from build123d import *

# Parameters (mm, degrees)
SKETCH1_W                 = 12
SKETCH1_H                 = 12
BOSS_EXTRUDE1_DEPTH       = 2
SKETCH2_W                 = 2.5
SKETCH2_H                 = 12
BOSS_EXTRUDE2_DEPTH       = 8
CUT_EXTRUDE1_DEPTH        = 17.733200531
CUT_EXTRUDE2_DEPTH        = 16.041608956
CUT_EXTRUDE2_DEPTH_BACK   = 16.041608956
SKETCH4_R                 = 2
SKETCH6_W                 = 5
SKETCH6_H                 = 3
BOSS_EXTRUDE3_DEPTH       = 10
F_3_0MM_DOWEL_HOLE1_D     = 3
F_3_0MM_DOWEL_HOLE1_DEPTH = 3
F_3_0MM_DOWEL_HOLE1_TIP   = 0.901290929


with BuildPart() as part:
    # Sketch1 → Boss-Extrude1 (new body)
    with BuildSketch(Plane(origin=(0, 0, 0), x_dir=(1, 0, 0), z_dir=(0, 1, 0))):
        Rectangle(SKETCH1_W, SKETCH1_H)
    extrude(amount=BOSS_EXTRUDE1_DEPTH)

    # Sketch2 → Boss-Extrude2 (add)
    with BuildSketch(Plane(origin=(0, 2, 0), x_dir=(1, 0, 0), z_dir=(0, 1, 0))):
        with Locations((-4.75, 0)):
            Rectangle(SKETCH2_W, SKETCH2_H)
        with Locations((4.75, 0)):
            Rectangle(SKETCH2_W, SKETCH2_H)
    extrude(amount=BOSS_EXTRUDE2_DEPTH)

    # Sketch5 → Cut-Extrude1 (cut, through all)
    with BuildSketch(Plane.XY.offset(6)):
        Polygon((-3.5, 10), (-6, 5.669872981), (-6, 10), align=None)
        Polygon((3.5, 10), (6, 5.669872981), (6, 10), align=None)
    extrude(amount=-CUT_EXTRUDE1_DEPTH, mode=Mode.SUBTRACT)

    # Sketch4 → Cut-Extrude2 (cut, two sides: drawn at the far end of the back side and taken through both)
    with BuildSketch(Plane.ZY.offset(-3.5).offset(-CUT_EXTRUDE2_DEPTH_BACK)):
        with Locations((0.326138493, 6)):
            Circle(SKETCH4_R)
    extrude(amount=CUT_EXTRUDE2_DEPTH + CUT_EXTRUDE2_DEPTH_BACK, mode=Mode.SUBTRACT)

    # Sketch6 → Boss-Extrude3 (add)
    with BuildSketch(Plane.XZ):
        with Locations((-3.5, -4.5)):
            Rectangle(SKETCH6_W, SKETCH6_H)
    extrude(amount=BOSS_EXTRUDE3_DEPTH)

    # Ø3.0mm Dowel Hole1
    with Locations(Plane.XY.offset(-3)):
        with Locations((-3.5, -5)):
            Hole(F_3_0MM_DOWEL_HOLE1_D / 2, depth=F_3_0MM_DOWEL_HOLE1_DEPTH)
            with Locations((0, 0, -(F_3_0MM_DOWEL_HOLE1_DEPTH + F_3_0MM_DOWEL_HOLE1_TIP / 2))):  # 118° drill point
                Cone(0, F_3_0MM_DOWEL_HOLE1_D / 2, F_3_0MM_DOWEL_HOLE1_TIP, mode=Mode.SUBTRACT)


solid = part.part
Build history of the part. All positions in model axes, mm. A direction names the side the tool comes from. Round coordinates to 2 decimals unless told otherwise and drop trailing zeros. Write each loop counter-clockwise with the first axis right and the second up, starting at its lowest first coordinate (ties: lowest second). Pieces come first, ordered by that corner, then holes. Notation, with made-up numbers: (87.25, 72) - (134.25, 72) arc R24 cw to (134.25, 103) - close; hole circle Ø8 at (77, 6.5). An arc over 180 degrees is marked (long way). One line per question, with ' | ' between items.
1. Drop flat-ended pins along their axis: pin 1 Ø2 at (y, z) = (7.5, 1) entering from -X; pin 2 Ø5.5 at (x, y) = (-3, -4) entering from +Z; pin 3 Ø5 at (y, z) = (-1.5, 0.5) entering from +X; pin 4 Ø2 at (x, z) = (-0.5, -2) entering from +Y. Give the stop position or say it passes through.
Results are:
pin 1: x = -5.13 | pin 2: z = -3 | pin 3: x = 6 | pin 4: y = 2
2. Band-saw the part on A-A, the plane y = -5. Write the cut outline in (x, z), and give its area (3 significant figures).
Results are:
outline: (-6, -6) - (-5, -6) - (-5, -3) - (-6, -3) - close; (-2, -6) - (-1, -6) - (-1, -3) - (-2, -3) - close | area: 6.00 mm^2
3. Drill centre lines: line 1 along X through (y, z) = (4, -0.5); line 2 along Z through (x, y) = (4.65, 6); line 3 along X through (y, z) = (-5, -5.1). Where is each one in solid material? Low to high. Write a range as from..to.
Results are:
line 1: -6..-3.5, 3.5..6 | line 2: -6..-1.67, 2.33..6 | line 3: -6..-5, -2..-1
4. Band-saw the part on B-B, the plane z = -4.75. Write the cut outline in (x, y).
Results are:
outline: (-6, -10) - (-1, -10) - (-1, 0) - (6, 0) - (6, 5.67) - (3.5, 10) - (3.5, 2) - (-3.5, 2) - (-3.5, 10) - (-6, 5.67) - close; hole circle Ø3 at (-3.5, -5)
5. Band-saw the part on D-D, the plane x = -2.75. Write the cut outline in (y, z), and give its area (3 significant figures).
Results are:
outline: (-10, -6) - (-6.3, -6) - (-6.3, -3) - (-10, -3) - close; (-3.7, -6) - (2, -6) - (2, 6) - (0, 6) - (0, -3) - (-3.7, -3) - close | area: 46.2 mm^2
6. Mould opens along Y. For faces 4 (the face through (4.455, 8.346, 0.084)), 5 (the face through (-0.1, 1.6, 6)), 6 (the face through (-4.45, 4.05, -0.11)) say: released by +Y, released by -Y, zero draft, split by the parting line, or undercut.
Results are:
face 4: released by +Y | face 5: zero draft | face 6: undercut
7. Band-saw the part on C-C, the plane y = 5.25. Write the cut outline in (x, z).
Results are:
outline: (-6, -6) - (-3.5, -6) - (-3.5, -1.53) - (-6, -1.53) - close; (-6, 2.18) - (-3.5, 2.18) - (-3.5, 6) - (-6, 6) - close; (3.5, -6) - (6, -6) - (6, -1.53) - (3.5, -1.53) - close; (3.5, 2.18) - (6, 2.18) - (6, 6) - (3.5, 6) - close
8. Tool access for faces 1 (the face through (-3.5, 4, -1)), 2 (the face through (-5, -4, -3)), 3 (the face through (-1, -5, -5)): list every direction of +Z, -Z, +X, -X, +Y, -Y with a clear straight run to the whole face (end or side of a thin tool).
Results are:
face 1: +Z, -Z, +Y | face 2: +Z, +X, -X, -Y | face 3: +Z, -Z, +X, -Y
